from build123d import *

# Parameters (mm, degrees)
SKETCH1_W           = 2000
SKETCH1_H           = 800
BOSS_EXTRUDE1_DEPTH = 12.7
SKETCH2_W           = 2000
SKETCH2_H           = 500
BOSS_EXTRUDE2_DEPTH = 200
SHELL1_START        = -187.3
SHELL1_OUTLINE_W    = 1974.6
SHELL1_OUTLINE_H    = 487.3
SHELL1_DEPTH        = 187.3
SKETCH4_W           = 25.4
SKETCH4_H           = 187.3
BOSS_EXTRUDE3_DEPTH = 487.3


# Read off the part's stored shape, not the designer's step: Shell1
with BuildPart() as part:
    # Sketch1 → Boss-Extrude1 (new body)
    with BuildSketch(Plane(origin=(0, 0, 0), x_dir=(1, 0, 0), z_dir=(0, 1, 0))):
        Rectangle(SKETCH1_W, SKETCH1_H)
    extrude(amount=BOSS_EXTRUDE1_DEPTH)

    # Sketch2 → Boss-Extrude2 (add)
    with BuildSketch(Plane.XZ):
        with Locations((0, -150)):
            Rectangle(SKETCH2_W, SKETCH2_H)
    extrude(amount=BOSS_EXTRUDE2_DEPTH)

    # Shell1 outline → Shell1 (cut)
    with BuildSketch(Plane(origin=(0, 0, 0), x_dir=(1, 0, 0), z_dir=(0, 1, 0)).offset(SHELL1_START)):
        with Locations((0, 143.65)):
            Rectangle(SHELL1_OUTLINE_W, SHELL1_OUTLINE_H)
    extrude(amount=SHELL1_DEPTH, mode=Mode.SUBTRACT)

    # Sketch4 → Boss-Extrude3 (add)
    with BuildSketch(Plane.XY.offset(-387.3)):
        with Locations((0, -93.65)):
            Rectangle(SKETCH4_W, SKETCH4_H)
    extrude(amount=BOSS_EXTRUDE3_DEPTH)


solid = part.part
Could you check a few things on this model? Use its own coordinates, in mm. A direction names the side the tool comes from. Round coordinates to 2 decimals unless told otherwise and drop trailing zeros. Order: outer loops, then holes, each group sorted by start corner. A loop starts at its lowest first (then second) coordinate and runs counter-clockwise, first axis right, second up.
(1) Imagine slicing it at D-D (z = 272.5). Write out the boundary of the cut face in (x, y), plus the area to 3 significant figures.
Response values:
outline: (-1000, 0) - (1000, 0) - (1000, 12.7) - (-1000, 12.7) - close
area: 25,400 mm2
(2) Which directions (+Z, -Z, +X, -X, +Y, -Y) give clear straight access to the entire face, cutting with the end or side of a thin tool? Please do faces 4 (the flat face through (-5, -159, 100)), 5 (the flat face through (-14, 0, 1)), 6 (the flat face through (1000, -92, -94)).
Response values:
face 4: +Z, +X, -X, -Y
face 5: +Z
face 6: +Z, -Z, +X, +Y, -Y
(3) Imagine slicing it at B-B (x = -438.5). Write out the boundary of the cut face in (y, z), plus the area to 3 significant figures.
Response values:
outline: (-200, -400) - (12.7, -400) - (12.7, 400) - (0, 400) - (0, -387.3) - (-187.3, -387.3) - (-187.3, 100) - (-200, 100) - close
area: 18,900 mm2
(4) Imagine slicing it at A-A (z = -263.5). Write out the boundary of the cut face in (x, y), plus the area to 3 significant figures.
Response values:
outline: (-1000, -200) - (1000, -200) - (1000, 12.7) - (-1000, 12.7) - close; hole (-987.3, -187.3) - (-12.7, -187.3) - (-12.7, 0) - (-987.3, 0) - close; hole (12.7, -187.3) - (987.3, -187.3) - (987.3, 0) - (12.7, 0) - close
area: 60,300 mm2
(5) If we mould it in two halves opening along Y, with no side actions, what happens to faces 1 (the flat face through (-14, 12.7, -6)), 2 (the flat face through (12.7, -95, -147)), 3 (the flat face through (-14, -200, -146))? For each: released by +Y, released by -Y, zero draft, split by the parting line, or undercut.
Response values:
face 1: released by +Y
face 2: undercut
face 3: released by -Y
(6) Imagine slicing it at C-C (y = -164.5). Write out the boundary of the cut face in (x, z).
Response values:
outline: (-1000, -400) - (1000, -400) - (1000, 100) - (987.3, 100) - (987.3, -387.3) - (12.7, -387.3) - (12.7, 100) - (-12.7, 100) - (-12.7, -387.3) - (-987.3, -387.3) - (-987.3, 100) - (-1000, 100) - close
(7) Please list where these lines run through material, in increasing order: line 1 along X through (y, z) = (-128, -91.5); line 2 along Y through (x, z) = (-254.5, 65.5); line 3 along Z through (x, y) = (544.5, -61).
Response values:
line 1: x = -1000 to -987.3, -12.7 to 12.7, 987.3 to 1000
line 2: y = -200 to -187.3, 0 to 12.7
line 3: z = -400 to -387.3
